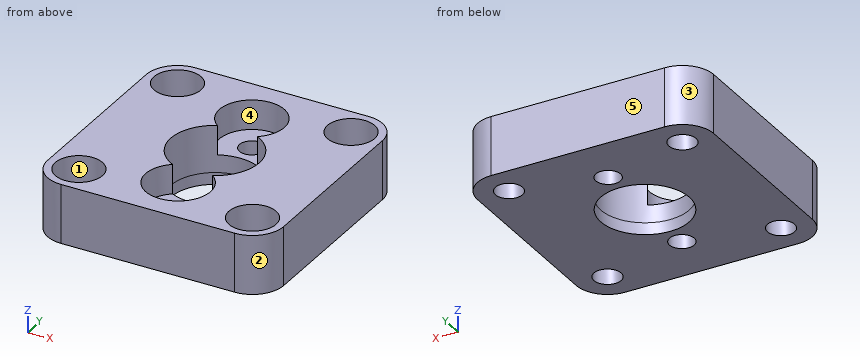
from build123d import *

# Parameters (mm, degrees)
SKIZZE3_W                       = 20
SKIZZE3_H                       = 20
SKIZZE3_R                       = 7.5
AUFSATZ_LINEAR_AUSTRAGEN2_DEPTH = 5
SKIZZE4_R                       = 1.05
SCHNITT_LINEAR_AUSTRAGEN1_DEPTH = 6
SKIZZE5_R                       = 2.75
SCHNITT_LINEAR_AUSTRAGEN2_DEPTH = 2.5
SCHNITT_LINEAR_AUSTRAGEN3_DEPTH = 6
SKIZZE7_R                       = 1.15
SCHNITT_LINEAR_AUSTRAGEN4_DEPTH = 6
SKIZZE8_R                       = 2
SCHNITT_LINEAR_AUSTRAGEN5_DEPTH = 3
SKIZZE10_R                      = 3.75
SCHNITT_LINEAR_AUSTRAGEN6_DEPTH = 6


with BuildPart() as part:
    # Skizze2 → Rotation1 (revolve)
    with BuildSketch(Plane(origin=(0, 0, 0), x_dir=(0, 0, -1), z_dir=(1, 0, 0))):
        Polygon((0, 3.75), (-1, 3.75), (-1, 3.25), (-2.6, 3.25), (-2.6, 2), (-5, 2), (-5, 7.5), (0, 7.5), align=None)
    revolve(axis=Axis((0, 0, 12.6), (0, 0, -1)))

    # Skizze3 → Aufsatz-Linear austragen2 (add, through all)
    with BuildSketch(Plane.XY.offset(5)):
        Rectangle(SKIZZE3_W, SKIZZE3_H)
        Circle(SKIZZE3_R, mode=Mode.SUBTRACT)
    extrude(amount=-AUFSATZ_LINEAR_AUSTRAGEN2_DEPTH)

    # Skizze4 → Schnitt-Linear austragen1 (cut, through all)
    with BuildSketch(Plane.XY.offset(5)):
        with Locations((0, 5.5)):
            Circle(SKIZZE4_R)
        with Locations((0, -5.5)):
            Circle(SKIZZE4_R)
    extrude(amount=-SCHNITT_LINEAR_AUSTRAGEN1_DEPTH, mode=Mode.SUBTRACT)

    # Skizze5 → Schnitt-Linear austragen2 (cut)
    with BuildSketch(Plane.XY.offset(5)):
        with Locations((0, 5.5)):
            Circle(SKIZZE5_R)
        with Locations((0, -5.5)):
            Circle(SKIZZE5_R)
    extrude(amount=-SCHNITT_LINEAR_AUSTRAGEN2_DEPTH, mode=Mode.SUBTRACT)

    # Skizze6 → Schnitt-Linear austragen3 (cut, through all)
    with BuildSketch(Plane.XY.offset(5)):
        with BuildLine():
            Line((-10, 7.352290732), (-10.887824638, 7.352290732))
            Line((-10.887824638, 7.352290732), (-10.887824638, 10.887824638))
            Line((-10.887824638, 10.887824638), (-7.352290732, 10.887824638))
            Line((-7.352290732, 10.887824638), (-7.352290732, 10))
            ThreePointArc((-7.352290732, 10), (-9.22450391, 9.22450391), (-10, 7.352290732))
        make_face()
        with BuildLine():
            Line((7.352290732, 10.887824638), (7.352290732, 10))
            ThreePointArc((7.352290732, 10), (9.22450391, 9.22450391), (10, 7.352290732))
            Line((10, 7.352290732), (10.887824638, 7.352290732))
            Line((10.887824638, 7.352290732), (10.887824638, 10.887824638))
            Line((10.887824638, 10.887824638), (7.352290732, 10.887824638))
        make_face()
        with BuildLine():
            Line((10, -7.352290732), (10.887824638, -7.352290732))
            Line((10.887824638, -7.352290732), (10.887824638, -10.887824638))
            Line((10.887824638, -10.887824638), (7.352290732, -10.887824638))
            Line((7.352290732, -10.887824638), (7.352290732, -10))
            ThreePointArc((7.352290732, -10), (9.22450391, -9.22450391), (10, -7.352290732))
        make_face()
        with BuildLine():
            Line((-7.352290732, -10.887824638), (-7.352290732, -10))
            ThreePointArc((-7.352290732, -10), (-9.22450391, -9.22450391), (-10, -7.352290732))
            Line((-10, -7.352290732), (-10.887824638, -7.352290732))
            Line((-10.887824638, -7.352290732), (-10.887824638, -10.887824638))
            Line((-10.887824638, -10.887824638), (-7.352290732, -10.887824638))
        make_face()
    extrude(amount=-SCHNITT_LINEAR_AUSTRAGEN3_DEPTH, mode=Mode.SUBTRACT)

    # Skizze7 → Schnitt-Linear austragen4 (cut, through all)
    with BuildSketch(Plane.XY.offset(5)):
        with Locations((-7.352290732, 7.352290732)):
            Circle(SKIZZE7_R)
        with Locations((7.352290732, 7.352290732)):
            Circle(SKIZZE7_R)
        with Locations((7.352290732, -7.352290732)):
            Circle(SKIZZE7_R)
        with Locations((-7.352290732, -7.352290732)):
            Circle(SKIZZE7_R)
    extrude(amount=-SCHNITT_LINEAR_AUSTRAGEN4_DEPTH, mode=Mode.SUBTRACT)

    # Skizze8 → Schnitt-Linear austragen5 (cut)
    with BuildSketch(Plane.XY.offset(5)):
        with Locations((-7.352290732, 7.352290732)):
            Circle(SKIZZE8_R)
        with Locations((7.352290732, 7.352290732)):
            Circle(SKIZZE8_R)
        with Locations((7.352290732, -7.352290732)):
            Circle(SKIZZE8_R)
        with Locations((-7.352290732, -7.352290732)):
            Circle(SKIZZE8_R)
    extrude(amount=-SCHNITT_LINEAR_AUSTRAGEN5_DEPTH, mode=Mode.SUBTRACT)

    # Skizze10 → Schnitt-Linear austragen6 (cut, through all)
    with BuildSketch(Plane(origin=(0, 0, 0), x_dir=(-1, 0, 0), z_dir=(0, 0, -1))):
        Circle(SKIZZE10_R)
    extrude(amount=-SCHNITT_LINEAR_AUSTRAGEN6_DEPTH, mode=Mode.SUBTRACT)


solid = part.part
Source: CAD feature listing. Evaluate the final solid. Frame: model axes, mm. Face numbers are marked on the shaded views. A direction names the side the tool comes from. Round coordinates to 2 decimals unless told otherwise and drop trailing zeros. Order: outer loops, then holes, each group sorted by start corner. A loop starts at its lowest first (then second) coordinate and runs counter-clockwise, first axis right, second up. Notation, with made-up numbers: (70, -39.5) - (81, -39.5) arc R12 cw to (81, -23.5) - close; hole circle Ø10 at (5.5, -8.75). An arc over 180 degrees is marked (long way). Use a Markdown table: item, result. Add a question column.
1. Set-up query: the marked faces 1 and 2. Return all of +Z, -Z, +X, -X, +Y, -Y with unobstructed straight access to the full face (end or side cutting, diameter ignored); none if empty.
2. Section query D-D (z = 1.6). Return the cut outline in (x, y), then the cut area to 3 significant figures.
3. Line query: probe 1 along Y at (x, z) = (0, 0.3); probe 2 along Y at (x, z) = (7.25, 1.45); probe 3 along X at (y, z) = (9, 2.7). Output: solid intervals per line, ascending.
4. First-contact query: pin 1 (4 mm diameter, centred on x = -0.5, y = -5, fed in from +Z); pin 2 (3.5 mm diameter, centred on x = -7.35, y = -7.35, fed in from +Z). Flat tips, straight axial feed; report the tip coordinate or a pass-through.
5. Section query A-A (y = 3). Return the cut outline in (x, z), then the cut area to 3 significant figures.
6. Section query B-B (x = 2). Return the cut outline in (y, z), then the cut area to 3 significant figures.
7. Mould query, pull axis X, two halves, no side actions, for the marked faces 3, 4 and 5. Classes: +X half, -X half, draft (parallel to the pull), parting line (faces both ways), or undercut.
8. Section query C-C (z = 4.6). Return the cut outline in (x, y).
Derived:
| question | item | result |
|---|---|---|
| 1 | face 1 | +Z |
| 1 | face 2 | +Z, -Z, +X, -Y |
| 2 | outline | (-10, -7.35) arc R2.65 ccw to (-7.35, -10) - (7.35, -10) arc R2.65 ccw to (10, -7.35) - (10, 7.35) arc R2.65 ccw to (7.35, 10) - (-7.35, 10) arc R2.65 ccw to (-10, 7.35) - close; hole circle Ø2.3 at (-7.35, -7.35); hole circle Ø2.3 at (-7.35, 7.35); hole circle Ø7.5 at (0, 0); hole circle Ø2.1 at (0, -5.5); hole circle Ø2.1 at (0, 5.5); hole circle Ø2.3 at (7.35, -7.35); hole circle Ø2.3 at (7.35, 7.35) |
| 2 | area | 326 mm2 |
| 3 | probe 1 | -10 to -6.55, -4.45 to -3.75, 3.75 to 4.45, 6.55 to 10 |
| 3 | probe 2 | -10 to -8.5, -6.21 to 6.21, 8.5 to 10 |
| 3 | probe 3 | -9.42 to -8.49, -6.22 to 6.22, 8.49 to 9.42 |
| 4 | pin 1 | z = 2.5 |
| 4 | pin 2 | z = 2 |
| 5 | outline | (-10, 0) - (-2.25, 0) - (-2.25, 5) - (-10, 5) - close; (2.25, 0) - (10, 0) - (10, 5) - (2.25, 5) - close |
| 5 | area | 77.5 mm2 |
| 6 | outline | (-10, 0) - (-3.17, 0) - (-3.17, 5) - (-3.61, 5) - (-3.61, 2.5) - (-7.39, 2.5) - (-7.39, 5) - (-10, 5) - close; (3.17, 0) - (10, 0) - (10, 5) - (7.39, 5) - (7.39, 2.5) - (3.61, 2.5) - (3.61, 5) - (3.17, 5) - close |
| 6 | area | 49.4 mm2 |
| 7 | face 3 | -X half |
| 7 | face 4 | undercut |
| 7 | face 5 | draft |
| 8 | outline | (-10, -7.35) arc R2.65 ccw to (-7.35, -10) - (7.35, -10) arc R2.65 ccw to (10, -7.35) - (10, 7.35) arc R2.65 ccw to (7.35, 10) - (-7.35, 10) arc R2.65 ccw to (-10, 7.35) - close; hole circle Ø4 at (-7.35, -7.35); hole circle Ø4 at (-7.35, 7.35); hole (-1.7, -3.34) arc R2.75 ccw (long way) to (1.7, -3.34) arc R3.75 ccw to (1.7, 3.34) arc R2.75 ccw (long way) to (-1.7, 3.34) arc R3.75 ccw to start; hole circle Ø4 at (7.35, -7.35); hole circle Ø4 at (7.35, 7.35) |
